```python
from build123d import *

# Parameters (mm, degrees)
F5_DEPTH        = 30
F7_DEPTH        = 27.5
F9_DEPTH        = 9.2
F11_DEPTH       = 9.2
F13_D           = 6.6
F13_CBORE_D     = 11.25
F13_CBORE_DEPTH = 27
F15_R           = 4
F16_DEPTH       = 39.001
F18_D           = 6.6
F18_CBORE_D     = 11.25
F18_CBORE_DEPTH = 2
F20_DEPTH       = 15
F22_D           = 6.6
F22_CBORE_D     = 11.25
F22_CBORE_DEPTH = 2
F24_DEPTH       = 3.001
F25_R           = 1.5
F25_R_2         = 12.5
F26_DEPTH       = 45.001
F28_D           = 3.4
F28_DEPTH       = 20
F28_CBORE_D     = 6.5
F28_CBORE_DEPTH = 3
F28_TIP         = 1.0214630523
F30_D           = 3.4
F30_DEPTH       = 20
F30_CBORE_D     = 6.5
F30_CBORE_DEPTH = 3
F30_TIP         = 1.0214630523
F31_SIZE        = 5


# Not quite as in the source:
# - a feature of the source that left no trace in its solid (it failed there, or was rolled back) is left out


with BuildPart() as f5:
    # F4 (on Front) → F5 (new body)
    with BuildSketch(Plane.XZ):
        Polygon((35, 46.5766017178), (7.5766017178, 74), (1.3633982822, 74), (-18.03, 54.6066017178), (-18.03, 43), (-43, 43), (-43, 0), (5, 0), (5, 30), (35, 30), align=None)
    extrude(amount=F5_DEPTH)

    # F6 (on face) → F7 (cut)
    with BuildSketch(Plane.XZ.offset(30)):
        Polygon((-43, 43), (-43, 0), (0, 0), (0, 30), (-18.03, 48.03), (-18.03, 43), align=None)
    extrude(amount=-F7_DEPTH, mode=Mode.SUBTRACT)

    # F8 (on offset) → F9 (cut)
    with BuildSketch(Plane.XZ.offset(14.1)):
        with BuildLine():
            Line((-18.03, 48.03), (-2.7734474577, 32.7734474577))
            Line((-2.7734474577, 32.7734474577), (9.5961081783, 47.0624990203))
            ThreePointArc((9.5961081783, 47.0624990203), (11.1595399436, 50.3961633531), (10.75, 54.0553864678))
            Line((10.75, 54.0553864678), (10.75, 70.8266017178))
            Line((10.75, 70.8266017178), (7.5766017178, 74))
            Line((7.5766017178, 74), (6.3357864376, 74))
            Line((6.3357864376, 74), (7.75, 72.5857864376))
            Line((7.75, 72.5857864376), (7.75, 61.4142135624))
            Line((7.75, 61.4142135624), (6.3357864376, 60))
            Line((6.3357864376, 60), (1.5055339059, 60))
            Line((1.5055339059, 60), (-5.5655339059, 67.0710678119))
            Line((-5.5655339059, 67.0710678119), (-18.03, 54.6066017178))
            Line((-18.03, 54.6066017178), (-18.03, 48.03))
        make_face()
    extrude(amount=-F9_DEPTH, mode=Mode.SUBTRACT)

    # F10 (on offset) → F11 (cut)
    with BuildSketch(Plane.XZ.offset(15.9)):
        with BuildLine():
            Line((1.3633982822, 74), (-16.6157864376, 56.0208152802))
            Line((-16.6157864376, 56.0208152802), (5.2500150699, 58.035865284))
            ThreePointArc((5.2500150699, 58.035865284), (10.7501324864, 60.7720041941), (12.97, 66.5))
            Line((12.97, 66.5), (12.97, 66.6066017178))
            Line((12.97, 66.6066017178), (14.97, 66.6066017178))
            Line((14.97, 66.6066017178), (7.5766017178, 74))
            Line((7.5766017178, 74), (1.3633982822, 74))
        make_face()
    extrude(amount=F11_DEPTH, mode=Mode.SUBTRACT)

    # F13 (through all)
    with Locations(Plane.XZ.offset(30)):
        with Locations((20, 45)):
            CounterBoreHole(F13_D / 2, F13_CBORE_D / 2, F13_CBORE_DEPTH)

    # F15 (on offset) → F16 (cut, through all)
    with BuildSketch(Plane(origin=(0, 0, 35), x_dir=(1, 0, 0), z_dir=(0, 0, -1))):
        with Locations((23.5, 15)):
            Circle(F15_R)
    extrude(amount=-F16_DEPTH, mode=Mode.SUBTRACT)

    # F18 (through all)
    with Locations(Plane(origin=(0, 0, 0), x_dir=(0, -1, 0), z_dir=(-1, 0, 0))):
        with Locations((16.25, 15)):
            CounterBoreHole(F18_D / 2, F18_CBORE_D / 2, F18_CBORE_DEPTH)

    # F19 (on face) → F20 (join)
    with BuildSketch(Plane.XZ.offset(30)):
        Polygon((5, 30), (35, 30), (35, 35), (35, 46.5766017178), (32, 49.5766017178), (32, 35), (5, 35), align=None)
    extrude(amount=F20_DEPTH)

    # F22 (through all)
    with Locations(Plane.XY.offset(35)):
        with Locations((18.5, -37.5)):
            CounterBoreHole(F22_D / 2, F22_CBORE_D / 2, F22_CBORE_DEPTH)

    # F23 (on face) → F24 (cut, through all)
    with BuildSketch(Plane(origin=(32, 0, 0), x_dir=(0, -1, 0), z_dir=(-1, 0, 0))):
        Polygon((45, 49.5766017178), (30, 49.5766017178), (45, 35), align=None)
    extrude(amount=-F24_DEPTH, mode=Mode.SUBTRACT)

    # F25 (on face) → F26 (cut, through all)
    with BuildSketch(Plane(origin=(0, 0, 0), x_dir=(-1, 0, 0), z_dir=(0, 1, 0))):
        with Locations((37, 37)):
            Circle(F25_R)
        with Locations((37, 6)):
            Circle(F25_R)
        with Locations((6, 6)):
            Circle(F25_R)
        with Locations((21.5, 21.5)):
            Circle(F25_R_2)
    extrude(amount=-F26_DEPTH, mode=Mode.SUBTRACT)

    # F28
    with Locations(Plane.XZ.offset(30)):
        with Locations((4.47, 66.5)):
            CounterBoreHole(F28_D / 2, F28_CBORE_D / 2, F28_CBORE_DEPTH, depth=F28_DEPTH)
            with Locations((0, 0, -(F28_DEPTH + F28_TIP / 2))):  # 118° drill point
                Cone(0, F28_D / 2, F28_TIP, mode=Mode.SUBTRACT)

    # F30
    with Locations(Plane(origin=(0, 0, 0), x_dir=(-1, 0, 0), z_dir=(0, 1, 0))):
        with Locations((-4.47, 51.5), (10.53, 51.5)):
            CounterBoreHole(F30_D / 2, F30_CBORE_D / 2, F30_CBORE_DEPTH, depth=F30_DEPTH)
            with Locations((0, 0, -(F30_DEPTH + F30_TIP / 2))):  # 118° drill point
                Cone(0, F30_D / 2, F30_TIP, mode=Mode.SUBTRACT)

    # F31
    f31_edges = [f5.edges().sort_by_distance(p)[0] for p in [
        (-18.03, -1.25, 43),
    ]]
    chamfer(f31_edges, length=F31_SIZE)


solid = f5.part
```
Part model, mm, in its own coordinate system. A direction names the side the tool comes from. Give positions to 0.01 mm unless a question says otherwise; leave off trailing zeros. Loops run counter-clockwise (first coordinate to the right, second up) from the corner with the lowest first, then second, coordinate; pieces in that order, holes last. Notation, with made-up numbers: M 43.25,-37.75 L 98.25,-37.75 A26 ccw 98.25,-7.75 Z; hole C -7.75,-12 d11. An arc over 180 degrees is marked long. Return JSON: item names as keys, results as strings.
1) Flat gauge pins, fed straight in: pin 1 Ø1.2 at (x, y) = (-31.5, -0.5) entering from +Z; pin 2 Ø8 at (y, z) = (-20, 46) entering from -X; pin 3 Ø3 at (x, y) = (-16.5, -27) entering from -Z. Where does each tip first touch, or does it go through?
Calculated:
{"pin 1": "stops at z = 43", "pin 2": "stops at x = -18.03", "pin 3": "stops at z = 45"}
2) Saw through at B-B, the plane x = -37. List the corners of the cut face in (y, z), then the cut area to 3 significant figures.
Calculated:
{"outline": "M -2.5,0 L 0,0 L 0,4.5 L -2.5,4.5 Z; M -2.5,7.5 L 0,7.5 L 0,35.5 L -2.5,35.5 Z; M -2.5,38.5 L 0,38.5 L 0,43 L -2.5,43 Z", "area": "92.5 mm2"}
3) 3-axis set-ups, long thin cutter, end or side, ignore diameter. For faces 4 (the face through (6, -27, 65)), 5 (the face through (-1, -25.1, 65)), 6 (the face through (22, -32, 35)), 7 (the face through (5, -28, 74)), 8 (the face through (-12, -3, 50)): which of +Z, -Z, +X, -X, +Y, -Y reach the whole face in a straight line?
Calculated:
{"face 4": "-Y", "face 5": "+Z, -X", "face 6": "+Z, -X, -Y", "face 7": "+Z, +X, -X, +Y, -Y", "face 8": "+Y"}
4) Saw through at A-A, the plane y = -23. List the corners of the cut face in (x, z) (3 decimals).
Calculated:
{"outline": "M -18.03,48.03 L 0,30 L 0,0 L 5,0 L 5,30 L 35,30 L 35,46.577 L 14.97,66.607 L 12.97,66.607 L 12.97,66.5 A8.5 cw 5.25,58.036 L -16.616,56.021 L -18.03,54.607 Z; hole C 20,45 d11.25"}
5) Pull direction Z, two halves, no side cores. Call faces 1 (the face through (10.75, -10, 62)), 2 (the face through (1, -12.1, 18.8)), 3 (the face through (21, -40, 33)): released by +Z, released by -Z, zero draft, split by the parting line, or undercut.
Calculated:
{"face 1": "zero draft", "face 2": "undercut", "face 3": "released by +Z"}
6) Saw through at D-D, the plane y = -29. List the corners of the cut face in (x, z) (3 decimals), then the cut area to 3 significant figures.
Calculated:
{"outline": "M -18.03,48.03 L 0,30 L 0,0 L 5,0 L 5,30 L 35,30 L 35,46.577 L 7.577,74 L 1.363,74 L -18.03,54.607 Z; hole C 4.47,66.5 d6.5; hole C 20,45 d11.25", "area": "1,620 mm2"}
7) Drill centre lines: line 1 (Z direction, x = 4.47, y = -29.4); line 2 (X direction, y = -11.15, z = 66.5); line 3 (Y direction, x = 18.5, z = 34.4) (3 decimals). Where is each one in solid material? Low to high.
Calculated:
{"line 1": "z = 0 to 63.25, 69.75 to 74", "line 2": "x = -4.99 to 2.77, 6.17 to 7.75, 10.75 to 15.08", "line 3": "y = -45 to -43.125, -31.875 to 0"}
8) Saw through at C-C, the plane z = 37. List the corners of the cut face in (x, y), then the cut area to 3 significant figures.
Calculated:
{"outline": "M -43,-2.5 L -38.5,-2.5 L -38.5,0 L -43,0 Z; M -35.5,-2.5 L -7,-2.5 L -7,-4.9 L 0.89,-4.9 L 0.89,-14.1 L -7,-14.1 L -7,-30 L 32,-30 L 32,-42.94 L 35,-42.94 L 35,0 L -35.5,0 Z; hole C 23.5,-15 d8", "area": "1,260 mm2"}
